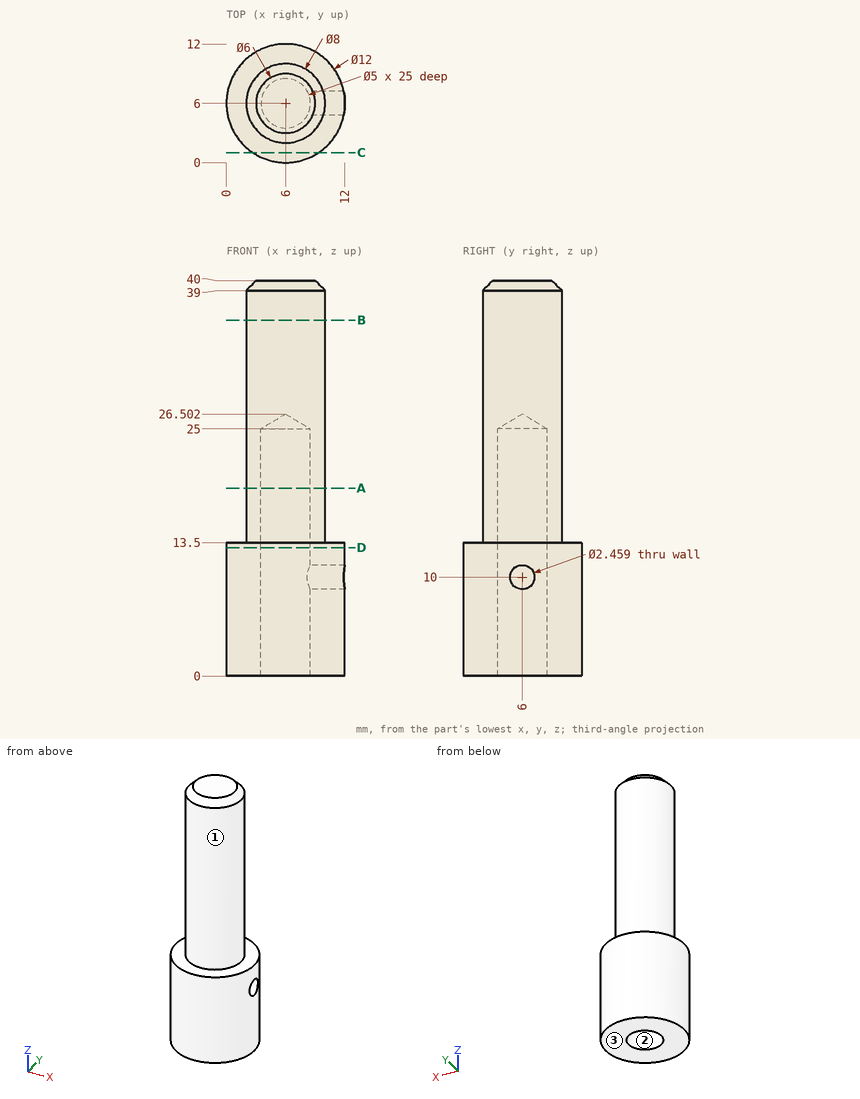
Job drawing, mm, ordinate dimensions from the low corner. One solid piece. Give positions to 0.01 mm unless a question says otherwise; leave off trailing zeros. Loops run counter-clockwise (first coordinate to the right, second up) from the corner with the lowest first, then second, coordinate; pieces in that order, holes last. Notation, with made-up numbers: (28.5, 49.5) -> (69.5, 49.5) arc R24 ccw to (69.5, 81.5) -> close; hole circle Ø10 at (-4, -16.5). An arc over 180 degrees is marked (long way). Write each question's results on one line, items separated by ' | '. Start each with the question number.
Q1. Pin check, flat tips, straight feed: P1, Ø2, axis at x = 10, z = 12, coming from the -Y side; P2, Ø5, axis at x = 11, z = 26.5, coming from the -Y side; P3, Ø1, axis at x = 6, z = 21.5, coming from the -Y side. Stop position of each tip, or through.
Q2. Band-saw the part on D-D on z = 13. List the corners of the cut face in (x, y).
Q3. Wall check: L1, parallel to Z at x = 8.5, y = 1.5; L2, parallel to Z at x = 10.5, y = 5.75; L3, parallel to X at y = 5.5, z = 15.5. Give the ranges that are in metal, low to high.
Q4. Band-saw the part on B-B on z = 36. List the corners of the cut face in (x, y).
Q5. Pull direction X, two halves, no side cores. Call the marked faces 1, 2 and 3: +X half, -X half, draft (parallel to the pull), parting line (faces both ways), or undercut.
Q6. Band-saw the part on C-C on y = 1. List the corners of the cut face in (x, z).
Q7. Band-saw the part on A-A on z = 19. List the corners of the cut face in (x, y), plus the area to 3 significant figures.
Results are:
1) P1: stops at y = 0.8 | P2: stops at y = 2.88 | P3: stops at y = 2
2) outline: circle Ø12 at (6, 6); hole circle Ø5 at (6, 6)
3) L1: z = 0 to 13.5 | L2: z = 0 to 8.8, 11.2 to 13.5 | L3: x = 2.03 to 3.55, 8.45 to 9.97
4) outline: circle Ø8 at (6, 6)
5) face 1: parting line | face 2: undercut | face 3: draft
6) outline: (2.68, 0) -> (9.32, 0) -> (9.32, 13.5) -> (2.68, 13.5) -> close
7) outline: circle Ø8 at (6, 6); hole circle Ø5 at (6, 6) | area: 30.6 mm²
